Part model, mm, in its own coordinate system. A direction names the side the tool comes from. Coordinates: 2 decimals unless noted, no trailing zeros. Write each loop counter-clockwise with the first axis right and the second up, starting at its lowest first coordinate (ties: lowest second). Pieces come first, ordered by that corner, then holes. Notation, with made-up numbers: (-30, -27.75) - (-6, -27.75) arc R5 cw to (-6, -20.75) - close; hole circle Ø11 at (-30.75, 19.5). An arc over 180 degrees is marked (long way). Write each question's results on one line, items separated by ' | '.
Solid Edge part; units mm, degrees
sketch "Sketch1" plane through (0, 0, 0) normal (0, 0, 1) x (1, 0, 0)
  circle A0 centre (0, 0) radius 10
extrude "Protrusion1" add sketch "Sketch1" along normal blind 14
sketch "Sketch2" plane through (0, 0, 0) normal (0, -1, 0) x (1, 0, 0)
  line L0 (10, 14.2715) -> (6, 14.2715)
  line L1 (6, 14.2715) -> (6, 8)
  line L2 (6, 8) -> (10, 8)
  line L3 (10, 8) -> (10, 14.2715)
  line L4 (6, 5.5) -> (6, 2.5)
  line L5 (6, 2.5) -> (10, 1)
  line L6 (10, 7) -> (10, 1)
  line L7 (6, 5.5) -> (10, 7)
  dimension "D1" = 6
revolve "RevolvedCutout1" cut sketch "Sketch2" angle 360 about axis through (0, 0, 0) along (0, 0, 1)
hole "Hole_1" at (0, 0, 14) direction (0, 0, -1) diameter 6 end through all
(1) Two-plate mould, pull along X, no slides. Class faces 4 (the flat face through (7, 0, 8)), 5 (the cylindrical face through (0, 3, 7)), 6 (the cylindrical face through (-2.17, 9.76, 0.49)): released by +X, released by -X, zero draft, split by the parting line, or undercut.
Return value:
face 4: zero draft | face 5: undercut | face 6: split by the parting line
(2) 3-axis set-ups, long thin cutter, end or side, ignore diameter. For faces 1 (the conical face through (-1.355, 6.102, 2.406)), 2 (the cylindrical face through (-6, 0, 11)), 3 (the flat face through (-3, -1, 14)): which of +Z, -Z, +X, -X, +Y, -Y reach the whole face in a straight line?
Return value:
face 1: none | face 2: +Z | face 3: +Z, +X, -X, +Y, -Y
(3) Saw through at C-C on z = 7.5. Write the cut outline in (x, y).
Return value:
outline: circle Ø20 at (0, 0); hole circle Ø6 at (0, 0)
(4) Flat gauge pin, fed straight in: P1, Ø3, axis at x = -6.5, y = -4.5, coming from the +Z side. Where does the tip first touch, or does it go through?
Return value:
P1: stops at z = 8
(5) Wall check: line 1 (X direction, y = 0, z = 9.75); line 2 (Y direction, x = -0.75, z = 3.25). Give the ranges that are in metal, low to high. Write a range as from..to.
Return value:
line 1: x = -6..-3, 3..6 | line 2: y = -5.95..-2.9, 2.9..5.95
(6) Saw through at A-A on x = 0. Write the cut outline in (y, z), then the cut area to 3 significant figures.
Return value:
outline: (-10, 0) - (-3, 0) - (-3, 14) - (-6, 14) - (-6, 8) - (-10, 8) - (-10, 7) - (-6, 5.5) - (-6, 2.5) - (-10, 1) - close; (3, 0) - (10, 0) - (10, 1) - (6, 2.5) - (6, 5.5) - (10, 7) - (10, 8) - (6, 8) - (6, 14) - (3, 14) - close | area: 112 mm^2
